Can you work these out from the model? Positions are in its coordinate system, mm. Face numbers are marked on the shaded views. A direction names the side the tool comes from. Coordinates: 2 decimals unless noted, no trailing zeros. Loops run counter-clockwise (first coordinate to the right, second up) from the corner with the lowest first, then second, coordinate; pieces in that order, holes last.
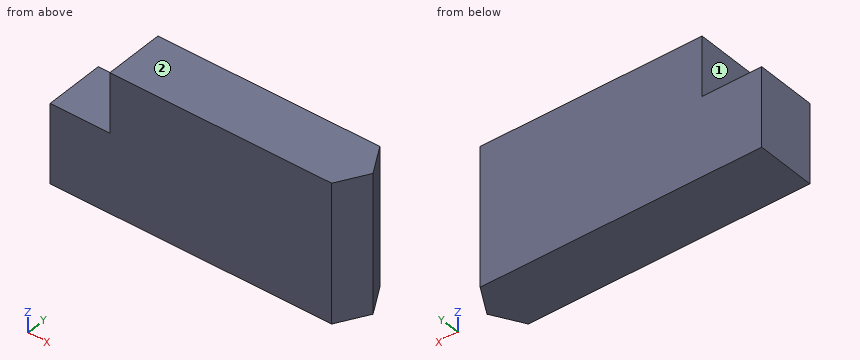
Autodesk Inventor part; units mm, degrees
ref_plane "YZ Plane" through (0, 0, 0) normal (1, 0, 0) x (0, 1, 0)
ref_plane "XZ Plane" through (0, 0, 0) normal (0, 1, 0) x (-1, 0, 0)
ref_plane "XY Plane" through (0, 0, 0) normal (0, 0, 1) x (1, 0, 0)
sketch "Sketch1" plane through (0, 0, 0) normal (0, 0, 1) x (1, 0, 0)
  line L0 (0, 0) -> (190.9559, 0)
  line L1 (190.9559, 0) -> (190.9559, 38.1)
  line L2 (190.9559, 38.1) -> (0, 38.1)
  line L3 (0, 38.1) -> (0, 0)
  dimension "d0" = 190.9559
  dimension "d1" = 38.1
extrude "Extrusion1" add sketch "Sketch1" along normal blind 88.9
sketch "Sketch2" plane through (0, 38.1, 0) normal (0, 1, 0) x (1, 0, 0)
  line L0 (0, -88.9) -> (190.9559, -88.9)
  line L1 (0, -88.9) -> (38.1, -88.9)
  line L2 (38.1, -88.9) -> (38.1, -50.8)
  line L3 (38.1, -50.8) -> (0, -50.8)
  line L4 (0, -50.8) -> (0, -88.9)
  point P0 (0, 0)
  dimension "d4" = 38.1
  dimension "d5" = 38.1
extrude "Extrusion2" cut sketch "Sketch2" against normal through all
sketch "Sketch4" plane through (0, 0, 88.9) normal (0, 0, 1) x (1, 0, 0)
  line L0 (190.9559, 38.1) -> (0, 38.1)
  line L1 (179.9574, 38.1) -> (190.9559, 19.05)
  line L2 (190.9559, 0) -> (190.9559, 38.1)
  line L3 (190.9559, 19.05) -> (179.9574, 0)
  line L4 (0, 0) -> (190.9559, 0)
  line L5 (179.9574, 0) -> (190.9559, 0)
  line L6 (190.9559, 0) -> (190.9559, 19.05)
  line L7 (190.9559, 38.1) -> (190.9559, 19.05)
  line L8 (179.9574, 38.1) -> (190.9559, 38.1)
  dimension "d12" = 60
  dimension "d13" = 60
extrude "Extrusion4" cut sketch "Sketch4" against normal through all
properties part number "BO04" material "Wood (Oak)"
Item 1: Suppose I cut it at D-D, the plane y = 34. Please give me the cut outline in (x, z).
Results are:
outline: (0, 0) - (182.32, 0) - (182.32, 88.9) - (38.1, 88.9) - (38.1, 50.8) - (0, 50.8) - close
Item 2: On a 3-axis mill with a long thin cutter (end or side, diameter ignored), from which of +Z, -Z, +X, -X, +Y, -Y can I reach the whole of each face in a straight line? I mean the marked faces 1 and 2. Say none if no direction works.
Results are:
face 1: +Z, -X, +Y, -Y
face 2: +Z, +X, -X, +Y, -Y
Item 3: Suppose I cut it at B-B, the plane y = 22. Please give me the cut outline in (x, z), plus the area to 3 significant figures.
Results are:
outline: (0, 0) - (189.25, 0) - (189.25, 88.9) - (38.1, 88.9) - (38.1, 50.8) - (0, 50.8) - close
area: 15,400 mm2
Item 4: Suppose I cut it at A-A, the plane z = 78. Please give me the cut outline in (x, y).
Results are:
outline: (38.1, 0) - (179.96, 0) - (190.96, 19.05) - (179.96, 38.1) - (38.1, 38.1) - close
Item 5: I'm going to push flat-ended pins straight in: P1, Ø5, axis at x = 63.5, y = 31.5, coming from the -Z side; P2, Ø11.5, axis at y = 27.5, z = 66, coming from the -X side; P3, Ø19, axis at x = 25.5, y = 22, coming from the +Z side. Where does each tip first touch, or does it pass through?
Results are:
P1: stops at z = 0
P2: stops at x = 38.1
P3: stops at z = 50.8
Item 6: I need wall thicknesses on line 1 along Z through (x, y) = (31, 35.5); line 2 along X through (y, z) = (22, 11); line 3 along X through (y, z) = (17.5, 14). Which ranges of each line are inside material? Lowest first, please.
Results are:
line 1: z = 0 to 50.8
line 2: x = 0 to 189.25
line 3: x = 0 to 190.06
Item 7: Suppose I cut it at C-C, the plane z = 31. Please give me the cut outline in (x, y).
Results are:
outline: (0, 0) - (179.96, 0) - (190.96, 19.05) - (179.96, 38.1) - (0, 38.1) - close
